```python
from build123d import *

# Parameters (mm, degrees)
EXTRUDE_1_DEPTH     = 5.3
SKETCH_2_OUTSIDE_W  = 61.562
SKETCH_2_OUTSIDE_H  = 63.574
SKETCH_2_OUTSIDE_R  = 6.25
CUT_EXTRUDE_1_DEPTH = 12.254924848
CUT_EXTRUDE_1_DRAFT = -60
SKETCH_3_R          = 4
EXTRUDE_2_DEPTH     = 40
CHAMFER_1_SIZE      = 1
FILLET_1_R          = 0.5


with BuildPart() as part:
    # Эскиз1 → Бобышка-Вытянуть1 (new body)
    with BuildSketch(Plane.XY):
        Polygon((0, 7.505553499), (-6.5, 3.75277675), (-6.5, -3.75277675), (0, -7.505553499), (6.5, -3.75277675), (6.5, 3.75277675), align=None)
    extrude(amount=EXTRUDE_1_DEPTH)


with BuildPart() as cut_extrude_1_tool:
    # Эскиз2 outside → Вырез-Вытянуть1 (with draft: the straight prism first)
    with BuildSketch(Plane.XY.offset(5.3)):
        Rectangle(SKETCH_2_OUTSIDE_W, SKETCH_2_OUTSIDE_H)
        Circle(SKETCH_2_OUTSIDE_R, mode=Mode.SUBTRACT)
    extrude(amount=-CUT_EXTRUDE_1_DEPTH)
    # Вырез-Вытянуть1: the draft: its side faces are tilted about the plane it starts from
    cut_extrude_1_sides = [cut_extrude_1_tool.faces().sort_by_distance(p)[0] for p in [
        (0, -31.787, -0.827462424),
        (30.781, 0, -0.827462424),
        (0, 31.787, -0.827462424),
        (-30.781, 0, -0.827462424),
        (-6.25, 0, -0.827462424),
    ]]
    draft(cut_extrude_1_sides, Plane.XY.offset(5.3), CUT_EXTRUDE_1_DRAFT)


with BuildPart() as part_1:
    add(part.part)

    # Вырез-Вытянуть1: cut by cut_extrude_1_tool
    add(cut_extrude_1_tool.part, mode=Mode.SUBTRACT)

    # Эскиз3 → Бобышка-Вытянуть2 (add)
    with BuildSketch(Plane(origin=(0, 0, 0), x_dir=(-1, 0, 0), z_dir=(0, 0, -1))):
        with Locations(Location((0, 0, 0), (0, 0, 180))):
            Circle(SKETCH_3_R)
    extrude(amount=EXTRUDE_2_DEPTH)

    # Фаска1
    chamfer_1_edges = [part_1.edges().sort_by_distance(p)[0] for p in [
        (-4, 0, -40),
    ]]
    chamfer(chamfer_1_edges, length=CHAMFER_1_SIZE)

    # Скругление1
    fillet_1_edges = [part_1.edges().sort_by_distance(p)[0] for p in [
        (-4, 0, 0),
    ]]
    fillet(fillet_1_edges, radius=FILLET_1_R)


solid = part_1.part
```
Part model, mm, in its own coordinate system. A direction names the side the tool comes from. Coordinates: 2 decimals unless noted, no trailing zeros. Order: outer loops, then holes, each group sorted by start corner. A loop starts at its lowest first (then second) coordinate and runs counter-clockwise, first axis right, second up. Notation, with made-up numbers: (-9.5, -14.5) -> (9.5, -14.5) arc R8 ccw to (9.5, -1.5) -> close; hole circle Ø2 at (42, 47.5). An arc over 180 degrees is marked (long way). Put each result on its own line as item: value. Start each with the question number.
(1) Band-saw the part on A-A (y = 0). Give the cut face in (x, z), then the cut area to 3 significant figures.
(2) Pin check, flat tips, straight feed: pin 1 Ø1.5 at (x, z) = (-3, -19.5) entering from +Y; pin 2 Ø1 at (x, y) = (1, 3.5) entering from -Z; pin 3 Ø3 at (y, z) = (0, -18.5) entering from +X. Stop position of each tip, or through.
(3) Band-saw the part on B-B (z = 2). Give the cut face in (x, y).
(4) Which spindle directions (+Z, -Z, +X, -X, +Y, -Y) get a long thin tool onto all of the face, cutting with end or side? Do faces 1 (the face through (3.2, -5.66, 2.54)), 2 (the face through (-4.4, -1.6, 0)). Say none if no direction does.
(5) Band-saw the part on C-C (z = -3). Give the cut face in (x, y).
(6) Probe line 1 along Z through (x, y) = (3.75, 4.5); line 2 along Y through (x, z) = (3, -6); line 3 along X through (y, z) = (-1.25, -19.5). List the from-to ranges inside material, lowest first. Write a range as [from, to].
Determined:
1. outline: (-6.5, 0) -> (-4.5, 0) arc R0.5 cw to (-4, -0.5) -> (-4, -39) -> (-3, -40) -> (3, -40) -> (4, -39) -> (4, -0.5) arc R0.5 cw to (4.5, 0) -> (6.5, 0) -> (6.5, 5.16) -> (6.25, 5.3) -> (-6.25, 5.3) -> (-6.5, 5.16) -> close
1. area: 388 mm²
2. pin 1: stops at y = 3.31
2. pin 2: stops at z = -39.86
2. pin 3: stops at x = 4
3. outline: (-6.5, -3.75) -> (0, -7.51) -> (6.5, -3.75) -> (6.5, 3.75) -> (0, 7.51) -> (-6.5, 3.75) -> close
4. face 1: +Z, -Z, +X, -Y
4. face 2: -Z
5. outline: circle Ø8 at (0, 0)
6. line 1: z = [0, 5.3]
6. line 2: y = [-2.65, 2.65]
6. line 3: x = [-3.8, 3.8]
